Could you check a few things on this model? Use its own coordinates, in mm. A direction names the side the tool comes from. Give positions to 0.01 mm unless a question says otherwise; leave off trailing zeros. Loops run counter-clockwise (first coordinate to the right, second up) from the corner with the lowest first, then second, coordinate; pieces in that order, holes last. Notation, with made-up numbers: (-14, -31.5) -> (15, -31.5) arc R33 cw to (15, -3.5) -> close; hole circle Ø10 at (44.25, 42.5). An arc over 180 degrees is marked (long way). Write each question's results on one line, items separated by ' | '. Start each with the question number.
Q1. If we section it at B-B, the plane x = -0.5: Give the number of separate pieces and of enclosed holes in the cut face, plus the area to 3 significant figures.
Q2. Which directions (+Z, -Z, +X, -X, +Y, -Y) give clear straight access to the entire face, cutting with the end or side of a thin tool? Please do faces 5 (the face through (0, -2.5, 0)), 6 (the face through (0, 0, -4.5)), 7 (the face through (1.014, 1.636, 8.211)), 8 (the face through (0, 0, 4.5)).
Q3. If we section it at A-A, the plane y = -1.35: List the corners of the cut face in (x, z) for me, plus the area to 3 significant figures.
Q4. If we section it at D-D, the plane y = 1.4: List the corners of the cut face in (x, z) for me.
Q5. Will these pins go through, and if not, where does the flat tip stop? P1, Ø1.2, axis at x = 0, y = 0, coming from the -Z side; P2, Ø1.2, axis at x = -0.5, y = 0, coming from the +Z side; P3, Ø1.8, axis at x = 0, y = 0, coming from the +Z side.
Q6. If I drill on line 1 along Z through (x, y) = (1.25, 0.2); line 2 along Y through (x, z) = (0, -5.25); line 3 along X through (y, z) = (0.75, 5.5), over which ranges is the centre line in solid material (lowest first)?
Q7. We'd pull the mould along Z, two halves only. Please class faces 1 (the face through (0, -1, 10)), 2 (the face through (2, -1, 8)), 3 (the face through (2.753, -0.345, 10.554)), 4 (the face through (0, -1.2, -11.5)): released by +Z, released by -Z, zero draft, split by the parting line, or undercut.
Autodesk Fusion 360 part; units mm, degrees
sketch "Sketch1" plane through (0, 0, 0) normal (0, 0, 1) x (1, 0, 0)
  line L0 (3, -2.5) -> (-3, -2.5)
  line L1 (-3, -2.5) -> (-3, 2.5)
  line L2 (-3, 2.5) -> (3, 2.5)
  line L3 (3, 2.5) -> (3, -2.5)
  line L4 (3, -2.5) -> (-3, 2.5) construction
  line L5 (-3, -2.5) -> (3, 2.5) construction
  dimension "dWidth" = 6
  dimension "d2" = 5
extrude "Extrude1" add sketch "Sketch1" along normal blind 11.5
sketch "Sketch2" plane through (0, 0, 11.5) normal (0, 0, 1) x (1, 0, 0)
  line L0 (3, 2.5) -> (-3, 2.5)
  line L1 (-3, 2.5) -> (-3, -2.5)
  line L2 (-3, -2.5) -> (3, -2.5)
  line L3 (3, -2.5) -> (3, 2.5)
  circle A0 centre (0, 0) radius 1
  dimension "d5" = 2
extrude "Extrude2" cut sketch "Sketch2" against normal blind 7 contours A0
ref_plane "WorkPlane1" through (0, 0, 9) normal (0, 0, 1) x (1, 0, 0)
sketch "Sketch3" plane through (0, 0, 9) normal (0, 0, 1) x (1, 0, 0)
  line L0 (2, -2.16) -> (-2, -2.16) construction
  line L1 (-2, -2.16) -> (-2, 2.16) construction
  line L2 (-2, 2.16) -> (2, 2.16) construction
  line L3 (2, 2.16) -> (2, -2.16) construction
  line L4 (2, -2.16) -> (-2, 2.16) construction
  line L5 (-2, -2.16) -> (2, 2.16) construction
  line L6 (-2, 0) -> (2, 0) construction
  line L7 (2, 1.1258) -> (2, -1.1258)
  line L8 (-2, 1.1258) -> (-2, -1.1258)
  line L9 (0, 2.16) -> (0, -2.16) construction
  line L10 (-2, 1.1258) -> (0, 2.16)
  line L11 (2, 1.1258) -> (0, 2.16)
  line L12 (-2, -1.1258) -> (0, -2.16) construction
  line L13 (0, -2.16) -> (2, -1.1258) construction
  line L14 (-2, -1.1258) -> (-2, -2.5)
  line L15 (-2, -2.5) -> (2, -2.5)
  line L16 (2, -2.5) -> (2, -1.1258)
  line L17 (3, -2.5) -> (-3, -2.5)
  dimension "d9" = 4
  dimension "d10" = 4.32
extrude "Extrude3" cut sketch "Sketch3" against normal blind 1.6
fillet "Fillet1" radius 0.75 2 edges at (-3, 2.5, 5.75) (3, 2.5, 5.75)
chamfer "Chamfer2" distance 0.5 angle 75 2 edges at (3, -0.375, 11.5) (-3, -0.375, 11.5) measured on face at (-2.3296, -0.2997, 11.5) measured on face at (-2.3296, -0.2997, 11.5)
mirror "Mirror2" about plane through (0, 0, 0) normal (0, 0, 1) of bodies 1 merged
properties part number "Configuration 2"
Final values:
1) separate pieces: 3 | enclosed holes: 0 | area: 81.3 mm²
2) face 5: +Z, -Z, +X, -X, -Y | face 6: -Z | face 7: -Y | face 8: +Z
3) outline: (-3, -9.63) -> (-2.5, -11.5) -> (2.5, -11.5) -> (3, -9.63) -> (3, 9.63) -> (2.5, 11.5) -> (-2.5, 11.5) -> (-3, 9.63) -> close; hole (-2, -9) -> (2, -9) -> (2, -7.4) -> (-2, -7.4) -> close; hole (-2, 7.4) -> (2, 7.4) -> (2, 9) -> (-2, 9) -> close | area: 123 mm²
4) outline: (-3, -9.63) -> (-2.5, -11.5) -> (2.5, -11.5) -> (3, -9.63) -> (3, 9.63) -> (2.5, 11.5) -> (-2.5, 11.5) -> (-3, 9.63) -> close; hole (-1.47, -9) -> (1.47, -9) -> (1.47, -7.4) -> (-1.47, -7.4) -> close; hole (-1.47, 7.4) -> (1.47, 7.4) -> (1.47, 9) -> (-1.47, 9) -> close
5) P1: stops at z = -4.5 | P2: stops at z = 11.5 | P3: stops at z = 4.5
6) line 1: z = -11.5 to -9, -7.4 to 7.4, 9 to 11.5 | line 2: y = -2.5 to -1, 1 to 2.5 | line 3: x = -3 to -0.66, 0.66 to 3
7) face 1: zero draft | face 2: undercut | face 3: released by +Z | face 4: released by -Z
